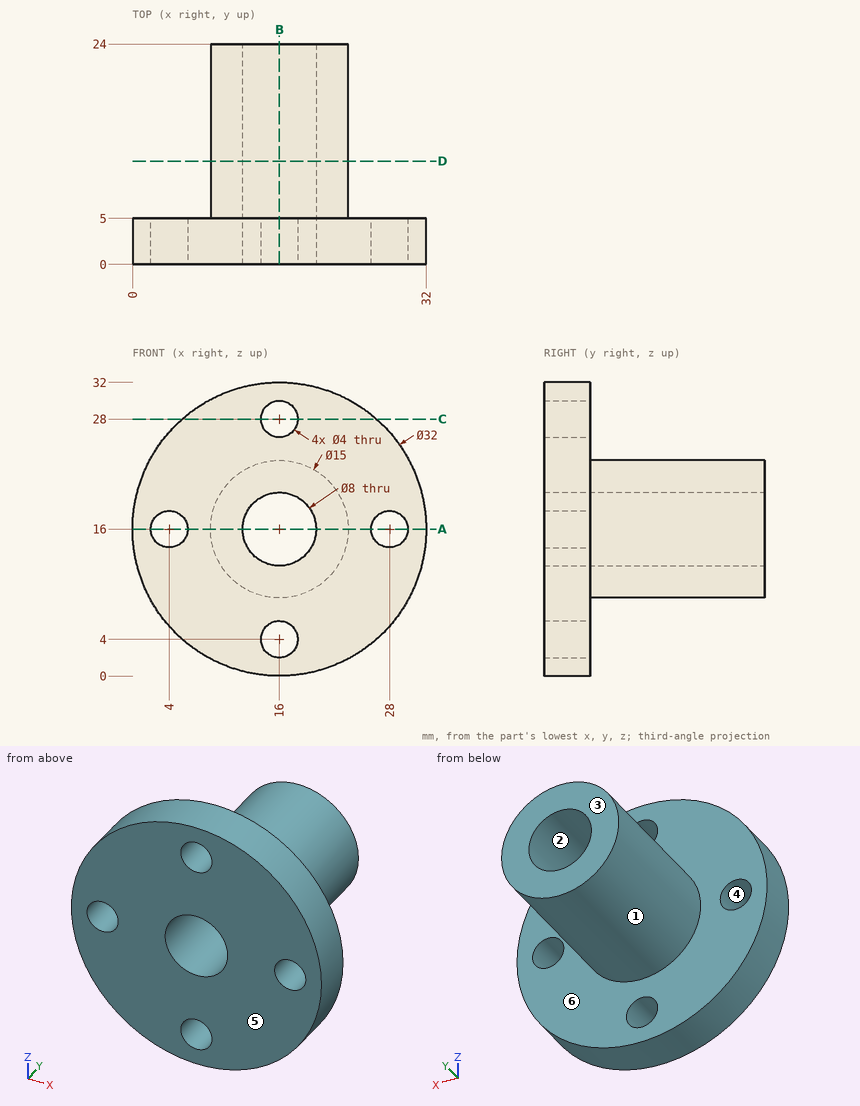
Here's the drawing with two shaded views (mm, measured from the low corner). I have some questions. A direction names the side the tool comes from. Coordinates: 2 decimals unless noted, no trailing zeros. Write each loop counter-clockwise with the first axis right and the second up, starting at its lowest first coordinate (ties: lowest second). Pieces come first, ordered by that corner, then holes. Notation, with made-up numbers: (-28, 52.5) -> (-17, 52.5) arc R30 ccw to (-17, 83.5) -> close; hole circle Ø11 at (-21.5, 31). An arc over 180 degrees is marked (long way). Use a Markdown table: item, result. Add a question column.
(1) If we section it at C-C, the plane z = 28: Write out the boundary of the cut face in (x, y), and give its area (3 significant figures).
(2) I'm going to push flat-ended pins straight in: P1, Ø3, axis at y = 8.5, z = 11.5, coming from the +X side; P2, Ø3, axis at x = 28, z = 16, coming from the +Y side; P3, Ø6, axis at x = 11.5, y = 17.5, coming from the +Z side; P4, Ø6, axis at x = 22, y = 6, coming from the -Z side. Where does each tip first touch, or does it pass through?
(3) If we section it at D-D, the plane y = 11.25: Write out the boundary of the cut face in (x, z), and give its area (3 significant figures).
(4) We'd pull the mould along Z, two halves only. Please class the marked faces 1, 2, 3 and 4: +Z half, -Z half, draft (parallel to the pull), parting line (faces both ways), or undercut.
(5) If we section it at A-A, the plane z = 16: Write out the boundary of the cut face in (x, y), and give its area (3 significant figures).
(6) If we section it at B-B, the plane x = 16: Write out the boundary of the cut face in (y, z), and give its area (3 significant figures).
(7) For the marked faces 5 and 6, which set-ups out of +Z, -Z, +X, -X, +Y, -Y let a thin tool reach every point of the face, with its end or its side?
(8) Please list where these lines run through material, in increasing order: line 1 (Z direction, x = 16, y = 2.65); line 2 (X direction, y = 19, z = 16).
Outcome:
| question | item | result |
|---|---|---|
| 1 | outline | (5.42, 0) -> (14, 0) -> (14, 5) -> (5.42, 5) -> close; (18, 0) -> (26.58, 0) -> (26.58, 5) -> (18, 5) -> close |
| 1 | area | 85.8 mm^2 |
| 2 | P1 | stops at x = 22.87 |
| 2 | P2 | passes through |
| 2 | P3 | stops at z = 23.35 |
| 2 | P4 | stops at z = 0.32 |
| 3 | outline | circle Ø15 at (16, 16); hole circle Ø8 at (16, 16) |
| 3 | area | 126 mm^2 |
| 4 | face 1 | parting line |
| 4 | face 2 | undercut |
| 4 | face 3 | draft |
| 4 | face 4 | undercut |
| 5 | outline | (0, 0) -> (2, 0) -> (2, 5) -> (0, 5) -> close; (6, 0) -> (12, 0) -> (12, 24) -> (8.5, 24) -> (8.5, 5) -> (6, 5) -> close; (20, 0) -> (26, 0) -> (26, 5) -> (23.5, 5) -> (23.5, 24) -> (20, 24) -> close; (30, 0) -> (32, 0) -> (32, 5) -> (30, 5) -> close |
| 5 | area | 213 mm^2 |
| 6 | outline | (0, 0) -> (5, 0) -> (5, 2) -> (0, 2) -> close; (0, 6) -> (5, 6) -> (5, 8.5) -> (24, 8.5) -> (24, 12) -> (0, 12) -> close; (0, 20) -> (24, 20) -> (24, 23.5) -> (5, 23.5) -> (5, 26) -> (0, 26) -> close; (0, 30) -> (5, 30) -> (5, 32) -> (0, 32) -> close |
| 6 | area | 213 mm^2 |
| 7 | face 5 | +Z, -Z, +X, -X, -Y |
| 7 | face 6 | +Y |
| 8 | line 1 | z = 0 to 2, 6 to 12, 20 to 26, 30 to 32 |
| 8 | line 2 | x = 8.5 to 12, 20 to 23.5 |
